from build123d import *

# Parameters (mm, degrees)
SKETCH_1_W          = 86
SKETCH_1_H          = 60
EXTRUDE_1_DEPTH     = 10
FILLET_1_R          = 3
SKETCH_2_R          = 1.25
CUT_EXTRUDE_1_DEPTH = 54.37602458
SKETCH_3_R          = 2.85
CUT_EXTRUDE_2_DEPTH = 3.1
SKETCH_4_R          = 1.75
CUT_EXTRUDE_3_DEPTH = 54.37602458


with BuildPart() as part:
    # 草图1 → 凸台-拉伸1 (new body)
    with BuildSketch(Plane(origin=(0, 0, 0), x_dir=(1, 0, 0), z_dir=(0, 1, 0))):
        Rectangle(SKETCH_1_W, SKETCH_1_H)
    extrude(amount=EXTRUDE_1_DEPTH)

    # 圆角1
    fillet_1_edges = [part.edges().sort_by_distance(p)[0] for p in [
        (43, 5, 30),
        (43, 5, -30),
    ]]
    fillet(fillet_1_edges, radius=FILLET_1_R)

    # 草图2 → 切除-拉伸1 (cut, through all)
    with BuildSketch(Plane(origin=(0, 10, 0), x_dir=(1, 0, 0), z_dir=(0, 1, 0))):
        with Locations(Location((-38, -8.88983487, 0), (0, 0, 270))):
            Circle(SKETCH_2_R)
        with Locations(Location((-38, 9.11016513, 0), (0, 0, 270))):
            Circle(SKETCH_2_R)
        with Locations(Location((0, 9, 0), (0, 0, 270))):
            Circle(SKETCH_2_R)
        with Locations(Location((0, -9, 0), (0, 0, 270))):
            Circle(SKETCH_2_R)
    extrude(amount=-CUT_EXTRUDE_1_DEPTH, mode=Mode.SUBTRACT)

    # 草图3 → 切除-拉伸2 (cut)
    with BuildSketch(Plane(origin=(0, 10, 0), x_dir=(1, 0, 0), z_dir=(0, 1, 0))):
        with Locations(Location((-38, -8.88983487, 0), (0, 0, 270))):
            Circle(SKETCH_3_R)
        with Locations(Location((-38, 9.11016513, 0), (0, 0, 270))):
            Circle(SKETCH_3_R)
        with Locations(Location((0, -9, 0), (0, 0, 270))):
            Circle(SKETCH_3_R)
        with Locations(Location((0, 9, 0), (0, 0, 270))):
            Circle(SKETCH_3_R)
    extrude(amount=-CUT_EXTRUDE_2_DEPTH, mode=Mode.SUBTRACT)

    # 草图4 → 切除-拉伸3 (cut, through all)
    with BuildSketch(Plane(origin=(0, 10, 0), x_dir=(1, 0, 0), z_dir=(0, 1, 0))):
        with Locations(Location((-22, -25, 0), (0, 0, 270))):
            Circle(SKETCH_4_R)
        with Locations(Location((-22, 25, 0), (0, 0, 270))):
            Circle(SKETCH_4_R)
        with Locations(Location((19, -25, 0), (0, 0, 270))):
            Circle(SKETCH_4_R)
        with Locations(Location((19, 25, 0), (0, 0, 270))):
            Circle(SKETCH_4_R)
    extrude(amount=-CUT_EXTRUDE_3_DEPTH, mode=Mode.SUBTRACT)


solid = part.part
CAD build for the part. Positions are in the model's coordinates, mm. A direction names the side the tool comes from. Give positions to 0.01 mm unless a question says otherwise; leave off trailing zeros. Order: outer loops, then holes, each group sorted by start corner. A loop starts at its lowest first (then second) coordinate and runs counter-clockwise, first axis right, second up. Notation, with made-up numbers: (1.25, 37.5) - (22.25, 37.5) arc R13 ccw to (22.25, 44.5) - close; hole circle Ø1 at (9.5, -29). An arc over 180 degrees is marked (long way). Write each question's results on one line, items separated by ' | '.
1. Pull direction X, two halves, no side cores. Call faces 1 (the face through (-2, 5, 30)), 2 (the face through (0.125, 8.472, 6.153)), 3 (the face through (42.1, 5.07, 29.14)): released by +X, released by -X, zero draft, split by the parting line, or undercut.
Calculated:
face 1: zero draft | face 2: undercut | face 3: released by +X
2. Saw through at A-A on z = 25. List the corners of the cut face in (x, y).
Calculated:
outline: (-43, 0) - (-23.75, 0) - (-23.75, 10) - (-43, 10) - close; (-20.25, 0) - (17.25, 0) - (17.25, 10) - (-20.25, 10) - close; (20.75, 0) - (43, 0) - (43, 10) - (20.75, 10) - close
3. Saw through at D-D on z = 9. List the corners of the cut face in (x, y), and give its area (3 significant figures).
Calculated:
outline: (-43, 0) - (-39.25, 0) - (-39.25, 6.9) - (-40.85, 6.9) - (-40.85, 10) - (-43, 10) - close; (-36.75, 0) - (-1.25, 0) - (-1.25, 6.9) - (-2.85, 6.9) - (-2.85, 10) - (-35.15, 10) - (-35.15, 6.9) - (-36.75, 6.9) - close; (1.25, 0) - (43, 0) - (43, 10) - (2.85, 10) - (2.85, 6.9) - (1.25, 6.9) - close | area: 790 mm2
4. Saw through at B-B on x = -22. List the corners of the cut face in (y, z).
Calculated:
outline: (0, -30) - (10, -30) - (10, -26.75) - (0, -26.75) - close; (0, -23.25) - (10, -23.25) - (10, 23.25) - (0, 23.25) - close; (0, 26.75) - (10, 26.75) - (10, 30) - (0, 30) - close
5. Probe L1, parallel to X at y = 4.5, z = -25; L2, parallel to X at y = 5.25, z = 9; L3, parallel to Z at x = 20, y = 7.5. List the from-to ranges inside material, lowest first. Write a range as from..to.
Calculated:
L1: x = -43..-23.75, -20.25..17.25, 20.75..43 | L2: x = -43..-39.25, -36.75..-1.25, 1.25..43 | L3: z = -30..-26.44, -23.56..23.56, 26.44..30
6. 3-axis set-ups, long thin cutter, end or side, ignore diameter. For faces 4 (the face through (-1, 10, 0)), 5 (the face through (-1, 6.9, 10)): which of +Z, -Z, +X, -X, +Y, -Y reach the whole face in a straight line?
Calculated:
face 4: +Z, -Z, +X, -X, +Y | face 5: +Y
7. Saw through at C-C on x = -38. List the corners of the cut face in (y, z), and give its area (3 significant figures).
Calculated:
outline: (0, -30) - (10, -30) - (10, -11.96) - (6.9, -11.96) - (6.9, -10.36) - (0, -10.36) - close; (0, -7.86) - (6.9, -7.86) - (6.9, -6.26) - (10, -6.26) - (10, 6.04) - (6.9, 6.04) - (6.9, 7.64) - (0, 7.64) - close; (0, 10.14) - (6.9, 10.14) - (6.9, 11.74) - (10, 11.74) - (10, 30) - (0, 30) - close | area: 530 mm2
8. Pin check, flat tip, straight feed: pin 1 (4 mm diameter, centred on x = 0, z = -9, fed in from +Y). Stop position of the tip, or through.
Calculated:
pin 1: stops at y = 6.9
